Autodesk Inventor part; units mm, degrees
ref_plane "YZ Plane" through (0, 0, 0) normal (1, 0, 0) x (0, 1, 0)
ref_plane "XZ Plane" through (0, 0, 0) normal (0, 1, 0) x (-1, 0, 0)
ref_plane "XY Plane" through (0, 0, 0) normal (0, 0, 1) x (1, 0, 0)
sketch "スケッチ1" plane through (0, 0, 0) normal (0, 0, 1) x (1, 0, 0)
  line L0 (8, -34) -> (-8, -34) construction
  arc A0 (-9.0607, -33.5607) -> (-8, -34) centre (-8, -32.5) ccw construction
  line L1 (-11.182, -31.4393) -> (-9.0607, -33.5607) construction
  arc A1 (-11.182, -31.4393) -> (-12.2426, -31) centre (-12.2426, -32.5) ccw construction
  line L2 (-30, -31) -> (-12.2426, -31) construction
  arc A2 (-33.0311, -29.25) -> (-30, -31) centre (-30, -27.5) ccw construction
  line L3 (-37.5311, -21.4558) -> (-33.0311, -29.25) construction
  arc A3 (-38, -19.7058) -> (-37.5311, -21.4558) centre (-34.5, -19.7058) ccw construction
  line L4 (-38, 13.5) -> (-38, -19.7058) construction
  arc A4 (-34.5, 17) -> (-38, 13.5) centre (-34.5, 13.5) ccw construction
  line L5 (34.5, 17) -> (-34.5, 17) construction
  arc A5 (38, 13.5) -> (34.5, 17) centre (34.5, 13.5) ccw construction
  line L6 (38, 13.5) -> (38, -19.7058) construction
  arc A6 (37.5311, -21.4558) -> (38, -19.7058) centre (34.5, -19.7058) ccw construction
  line L7 (37.5311, -21.4558) -> (33.0311, -29.25) construction
  arc A7 (30, -31) -> (33.0311, -29.25) centre (30, -27.5) ccw construction
  line L8 (30, -31) -> (12.2426, -31) construction
  arc A8 (12.2426, -31) -> (11.182, -31.4393) centre (12.2426, -32.5) ccw construction
  line L9 (11.182, -31.4393) -> (9.0607, -33.5607) construction
  arc A9 (8, -34) -> (9.0607, -33.5607) centre (8, -32.5) ccw construction
  line L10 (32.8579, -29.15) -> (37.3579, -21.3558)
  arc A10 (37.3579, -21.3558) -> (37.8, -19.7058) centre (34.5, -19.7058) ccw
  line L11 (37.8, -19.7058) -> (37.8, 13.5)
  arc A11 (37.8, 13.5) -> (34.5, 16.8) centre (34.5, 13.5) ccw
  line L12 (34.5, 16.8) -> (-34.5, 16.8)
  arc A12 (-34.5, 16.8) -> (-37.8, 13.5) centre (-34.5, 13.5) ccw
  line L13 (-37.8, 13.5) -> (-37.8, -19.7058)
  arc A13 (-37.8, -19.7058) -> (-37.3579, -21.3558) centre (-34.5, -19.7058) ccw
  line L14 (-37.3579, -21.3558) -> (-32.8579, -29.15)
  arc A14 (-32.8579, -29.15) -> (-30, -30.8) centre (-30, -27.5) ccw
  line L15 (-30, -30.8) -> (-12.2426, -30.8)
  arc A15 (-11.0406, -31.2979) -> (-12.2426, -30.8) centre (-12.2426, -32.5) ccw
  line L16 (-11.0406, -31.2979) -> (-8.9192, -33.4192)
  arc A16 (-8.9192, -33.4192) -> (-8, -33.8) centre (-8, -32.5) ccw
  line L17 (-8, -33.8) -> (8, -33.8)
  arc A17 (8, -33.8) -> (8.9192, -33.4192) centre (8, -32.5) ccw
  line L18 (8.9192, -33.4192) -> (11.0406, -31.2979)
  arc A18 (12.2426, -30.8) -> (11.0406, -31.2979) centre (12.2426, -32.5) ccw
  line L19 (12.2426, -30.8) -> (30, -30.8)
  arc A19 (30, -30.8) -> (32.8579, -29.15) centre (30, -27.5) ccw
  circle A20 centre (-13, -26) radius 1.1
  circle A21 centre (-13, 14) radius 1.1
  arc A22 (-13, -23) -> (-16, -26) centre (-13, -26) ccw construction
  arc A23 (-16, 14) -> (-13, 11) centre (-13, 14) ccw construction
  line L20 (0, 0) -> (0, -37.0919) construction
  circle A24 centre (13, -26) radius 1.1
  circle A25 centre (13, 14) radius 1.1
  dimension "d28" = 0.2
  dimension "d29" = 2.2
extrude "押し出し1" add sketch "スケッチ1" against normal blind 1.6
properties part number "main_pcb" material "GFRC"
Could you check a few things on this model? Use its own coordinates, in mm. A direction names the side the tool comes from. Give positions to 0.01 mm unless a question says otherwise; leave off trailing zeros. Order: outer loops, then holes, each group sorted by start corner. A loop starts at its lowest first (then second) coordinate and runs counter-clockwise, first axis right, second up.
Item 1: If we section it at A-A, the plane x = 13: Write out the boundary of the cut face in (y, z), plus the area to 3 significant figures.
Item 2: If we mould it in two halves opening along X, with no side actions, what happens to faces 1 (the face through (-36.808, 15.859, -0.789)), 2 (the face through (21, -30.8, -1)), 3 (the face through (12.762, 12.926, -0.789))? For each: pulls with the +X half, pulls with the -X half, needs draft (parallel to the pull), parting line crosses it, or undercut.
Item 3: For faces 4 (the face through (-21, -30.8, -1)), 5 (the face through (36.859, 15.808, -0.789)), which set-ups out of +Z, -Z, +X, -X, +Y, -Y let a thin tool reach every point of the face, with its end or its side?
Item 4: I need wall thicknesses on line 1 (Y direction, x = -13, z = -0.8); line 2 (X direction, y = -27, z = -0.5); line 3 (X direction, y = 13, z = -0.7). Which ranges of each line are inside material? Lowest first, please.
Item 5: If we section it at B-B, the plane y = -26: Write out the boundary of the cut face in (x, z).
Item 6: If we section it at C-C, the plane z = -0.6: Write out the boundary of the cut face in (x, y).
Item 7: I'm going to push flat-ended pins straight in: pin 1 (0.8 mm diameter, centred on x = 17, z = -0.5, fed in from -Y); pin 2 (1.8 mm diameter, centred on x = -13, y = 14, fed in from -Z). Where does each tip first touch, or does it pass through?
Item 8: If we section it at D-D, the plane x = -23.5: Write out the boundary of the cut face in (y, z).
Values:
1. outline: (-30.8, -1.6) - (-27.1, -1.6) - (-27.1, 0) - (-30.8, 0) - close; (-24.9, -1.6) - (12.9, -1.6) - (12.9, 0) - (-24.9, 0) - close; (15.1, -1.6) - (16.8, -1.6) - (16.8, 0) - (15.1, 0) - close
1. area: 69.1 mm2
2. face 1: pulls with the -X half
2. face 2: needs draft
2. face 3: undercut
3. face 4: +Z, -Z, -X, -Y
3. face 5: +Z, -Z, +X, +Y
4. line 1: y = -30.8 to -27.1, -24.9 to 12.9, 15.1 to 16.8
4. line 2: x = -34.1 to -13.46, -12.54 to 12.54, 13.46 to 34.1
4. line 3: x = -37.8 to -13.46, -12.54 to 12.54, 13.46 to 37.8
5. outline: (-34.68, -1.6) - (-14.1, -1.6) - (-14.1, 0) - (-34.68, 0) - close; (-11.9, -1.6) - (11.9, -1.6) - (11.9, 0) - (-11.9, 0) - close; (14.1, -1.6) - (34.68, -1.6) - (34.68, 0) - (14.1, 0) - close
6. outline: (-37.8, -19.71) arc R3.3 ccw to (-37.36, -21.36) - (-32.86, -29.15) arc R3.3 ccw to (-30, -30.8) - (-12.24, -30.8) arc R1.7 cw to (-11.04, -31.3) - (-8.92, -33.42) arc R1.3 ccw to (-8, -33.8) - (8, -33.8) arc R1.3 ccw to (8.92, -33.42) - (11.04, -31.3) arc R1.7 cw to (12.24, -30.8) - (30, -30.8) arc R3.3 ccw to (32.86, -29.15) - (37.36, -21.36) arc R3.3 ccw to (37.8, -19.71) - (37.8, 13.5) arc R3.3 ccw to (34.5, 16.8) - (-34.5, 16.8) arc R3.3 ccw to (-37.8, 13.5) - close; hole circle Ø2.2 at (-13, -26); hole circle Ø2.2 at (-13, 14); hole circle Ø2.2 at (13, -26); hole circle Ø2.2 at (13, 14)
7. pin 1: stops at y = -30.8
7. pin 2: passes through
8. outline: (-30.8, -1.6) - (16.8, -1.6) - (16.8, 0) - (-30.8, 0) - close
